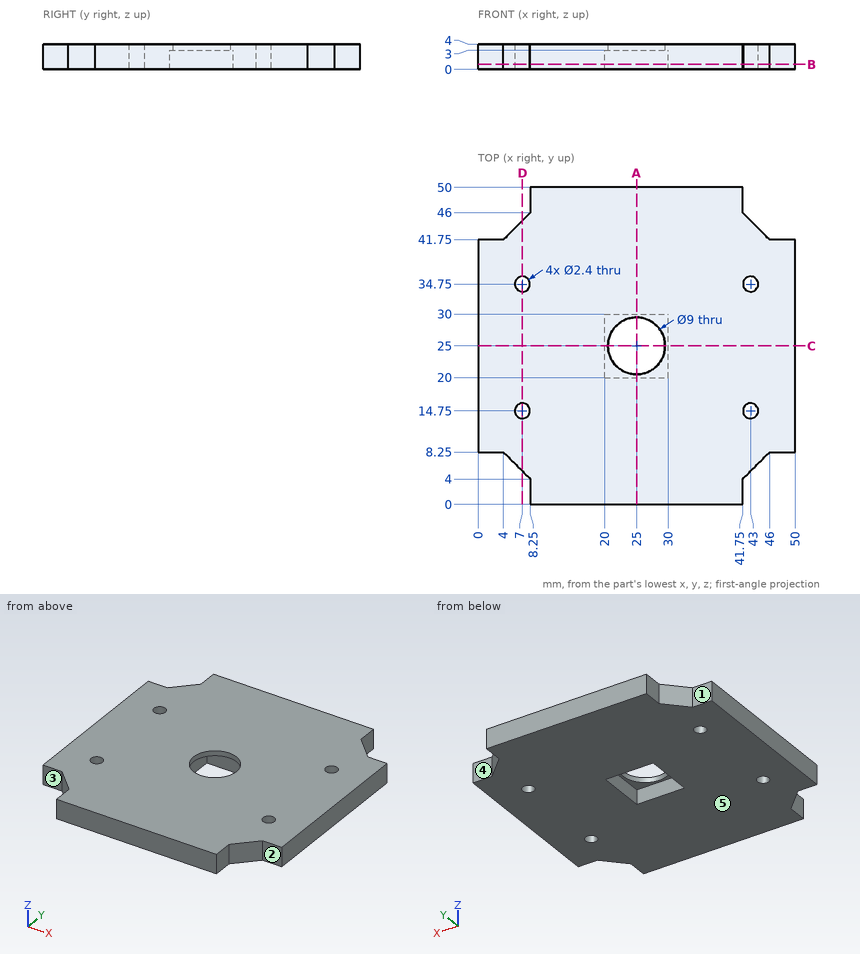
The figure shows three views and two pictorial views of one solid part (mm, origin at its lowest corner). Answer the questions. A direction names the side the tool comes from. Round coordinates to 2 decimals unless told otherwise and drop trailing zeros. Order: outer loops, then holes, each group sorted by start corner. A loop starts at its lowest first (then second) coordinate and runs counter-clockwise, first axis right, second up. Notation, with made-up numbers: (-32.5, 8.5) - (-16.5, 8.5) arc R21 ccw to (-16.5, 41.5) - close; hole circle Ø9 at (35, -34). An arc over 180 degrees is marked (long way). Write item = value, one per line. Start each with the question number.
1) For the marked faces 1, 2, 3, 4 and 5, determine the directions among +Z, -Z, +X, -X, +Y, -Y from which every point of the face is accessible in a straight line to the end or side of a thin tool.
2) Section D-D, the plane x = 7 is taken. Write down the section's boundary in (y, z).
3) Straight lines are drawn through the part: L1, parallel to X at y = 25, z = 3.2; L2, parallel to Y at x = 6, z = 1.1; L3, parallel to X at y = 29, z = 2.45. For each, find the intervals that lie inside material, in ascending order.
4) Given pin 1 (1 mm diameter, centred on x = 43, z = 3.5, fed in from +Y); pin 2 (1.2 mm diameter, centred on y = 47, z = 1, fed in from -X); pin 3 (1.4 mm diameter, centred on x = 7, y = 14.75, fed in from -Z); pin 4 (2 mm diameter, centred on y = 47.5, z = 2.5, fed in from +X), each flat-ended and moving along its own axis, determine where each tip first touches the part or whether it passes through.
5) Section B-B, the plane z = 0.8 is taken. Write down the section's boundary in (x, y), plus the area to 3 significant figures.
6) Section A-A, the plane x = 25 is taken. Write down the section's boundary in (y, z), plus the area to 3 significant figures.
Results list:
q1.face_1 = +Z, -Z, -X, +Y
q1.face_2 = +Z, -Z, +X, -Y
q1.face_3 = +Z, -Z, -X, -Y
q1.face_4 = +Z, -Z, +X, +Y
q1.face_5 = -Z, +X, -X, +Y, -Y
q2.outline = (5.25, 0) - (13.55, 0) - (13.55, 4) - (5.25, 4) - close; (15.95, 0) - (33.55, 0) - (33.55, 4) - (15.95, 4) - close; (35.95, 0) - (44.75, 0) - (44.75, 4) - (35.95, 4) - close
q3.L1 = 0 to 20.5, 29.5 to 50
q3.L2 = 6.25 to 14.09, 15.41 to 34.09, 35.41 to 43.75
q3.L3 = 0 to 20, 30 to 50
q4.pin_1 = 45.25
q4.pin_2 = 8.25
q4.pin_3 = through
q4.pin_4 = 41.75
q5.outline = (0, 8.25) - (4, 8.25) - (8.25, 4) - (8.25, 0) - (41.75, 0) - (41.75, 4) - (46, 8.25) - (50, 8.25) - (50, 41.75) - (46, 41.75) - (41.75, 46) - (41.75, 50) - (8.25, 50) - (8.25, 46) - (4, 41.75) - (0, 41.75) - close; hole circle Ø2.4 at (7, 14.75); hole circle Ø2.4 at (7, 34.75); hole (20, 20) - (30, 20) - (30, 30) - (20, 30) - close; hole circle Ø2.4 at (43, 14.75); hole circle Ø2.4 at (43, 34.75)
q5.area = 2,150 mm^2
q6.outline = (0, 0) - (20, 0) - (20, 3) - (20.5, 3) - (20.5, 4) - (0, 4) - close; (29.5, 3) - (30, 3) - (30, 0) - (50, 0) - (50, 4) - (29.5, 4) - close
q6.area = 161 mm^2
